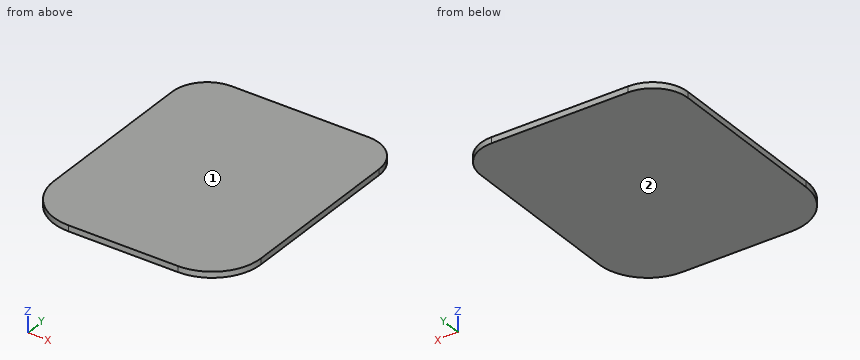
```python
from build123d import *

# Parameters (mm, degrees)
BOSS_EXTRUDE1_DEPTH = 4.3


with BuildPart() as part:
    # Sketch1 → Boss-Extrude1 (new body)
    with BuildSketch(Plane.XY):
        with BuildLine():
            Line((0.5, -92.2), (40, -92.2))
            ThreePointArc((40, -92.2), (65.243712088, -81.743712088), (75.7, -56.5))
            Line((75.7, -56.5), (75.7, 66.5))
            ThreePointArc((75.7, 66.5), (68.172644276, 84.672644276), (50, 92.2))
            Line((50, 92.2), (-50, 92.2))
            ThreePointArc((-50, 92.2), (-68.172644276, 84.672644276), (-75.7, 66.5))
            Line((-75.7, 66.5), (-75.7, -56.5))
            ThreePointArc((-75.7, -56.5), (-65.243712088, -81.743712088), (-40, -92.2))
            Line((-40, -92.2), (-0.5, -92.2))
            Line((-0.5, -92.2), (0.5, -92.2))
        make_face()
    extrude(amount=BOSS_EXTRUDE1_DEPTH)


solid = part.part
```
Could you check a few things on this model? Use its own coordinates, in mm. Face numbers are marked on the shaded views. Coordinates: 2 decimals unless noted, no trailing zeros. Loops run counter-clockwise (first coordinate to the right, second up) from the corner with the lowest first, then second, coordinate; pieces in that order, holes last.
1) Please list where these lines run through material, in increasing order: line 1 along Y through (x, z) = (49.5, 2.3); line 2 along Y through (x, z) = (55.5, 2.3); line 3 along X through (y, z) = (85, 3.2).
Reported:
line 1: y = -90.91 to 92.2
line 2: y = -88.66 to 91.6
line 3: x = -67.84 to 67.84
2) Will this pin go through, and if not, where does the flat tip stop? pin 1 Ø1.5 at (x, y) = (46, -63.5) entering from -Z.
Reported:
pin 1: stops at z = 0
3) Imagine slicing it at B-B (x = 61.5). List the corners of the cut face in (y, z) for me.
Reported:
outline: (-85, 0) - (89.48, 0) - (89.48, 4.3) - (-85, 4.3) - close
4) Thinking about a two-plate mould opening in Z: for the marked faces 1 and 2, which applies, released by +Z, released by -Z, zero draft, split by the parting line, or undercut?
Reported:
face 1: released by +Z
face 2: released by -Z
5) Imagine slicing it at C-C (y = -69). List the corners of the cut face in (x, z) for me, and give its area (3 significant figures).
Reported:
outline: (-73.44, 0) - (73.44, 0) - (73.44, 4.3) - (-73.44, 4.3) - close
area: 632 mm2
6) Imagine slicing it at A-A (z = 1). List the corners of the cut face in (x, y) for me.
Reported:
outline: (-75.7, -56.5) arc R35.7 ccw to (-40, -92.2) - (40, -92.2) arc R35.7 ccw to (75.7, -56.5) - (75.7, 66.5) arc R25.7 ccw to (50, 92.2) - (-50, 92.2) arc R25.7 ccw to (-75.7, 66.5) - close
